```python
from build123d import *

# Parameters (mm, degrees)
SKETCH1_R           = 0.9
BOSS_EXTRUDE1_DEPTH = 5
SKETCH2_R           = 2.5
BOSS_EXTRUDE2_DEPTH = 1
DOME1_FACE_RADIUS   = 2.5
DOME1_HEIGHT        = 0.5
SKETCH3_W           = 1.125
SKETCH3_H           = 0.75
SKETCH3_W_2         = 0.75
SKETCH3_H_2         = 1.125
CUT_EXTRUDE1_DEPTH  = 0.75


with BuildPart() as part:
    # Sketch1 → Boss-Extrude1 (new body)
    with BuildSketch(Plane(origin=(0, 0, 0), x_dir=(1, 0, 0), z_dir=(0, 1, 0))):
        Circle(SKETCH1_R)
    extrude(amount=BOSS_EXTRUDE1_DEPTH)

    # Sketch2 → Boss-Extrude2 (add)
    with BuildSketch(Plane(origin=(0, 5, 0), x_dir=(1, 0, 0), z_dir=(0, 1, 0))):
        Circle(SKETCH2_R)
    extrude(amount=BOSS_EXTRUDE2_DEPTH)

    # Dome1: a dome of height H over a round flat face of radius A is a cap of a sphere of radius (A * A + H * H) / (2 * H)
    dome1_r = (DOME1_FACE_RADIUS * DOME1_FACE_RADIUS + DOME1_HEIGHT * DOME1_HEIGHT) / (2 * DOME1_HEIGHT)
    dome1_base = Plane((0, 6, 0), z_dir=(0, 1, 0))
    with Locations(dome1_base.offset(DOME1_HEIGHT - dome1_r)):
        dome1_ball = Sphere(dome1_r, mode=Mode.PRIVATE)
    add(split(dome1_ball, bisect_by=dome1_base, keep=Keep.TOP, mode=Mode.PRIVATE))

    # Sketch3 → Cut-Extrude1 (cut)
    with BuildSketch(Plane(origin=(0, 6.5, 0), x_dir=(1, 0, 0), z_dir=(0, 1, 0))):
        with Locations((-0.9375, 0)):
            Rectangle(SKETCH3_W, SKETCH3_H)
        Rectangle(SKETCH3_W_2, SKETCH3_H)
        with Locations((0, 0.9375)):
            Rectangle(SKETCH3_W_2, SKETCH3_H_2)
        with Locations((0.9375, 0)):
            Rectangle(SKETCH3_W, SKETCH3_H)
        with Locations((0, -0.9375)):
            Rectangle(SKETCH3_W_2, SKETCH3_H_2)
    extrude(amount=-CUT_EXTRUDE1_DEPTH, mode=Mode.SUBTRACT)


solid = part.part
```
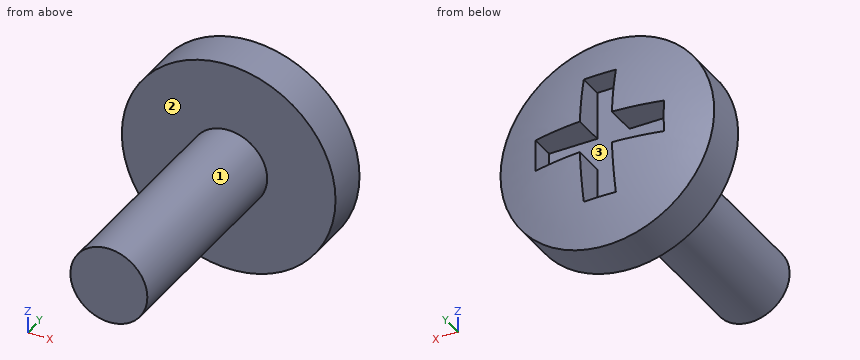
Geometry: final body of the model. Coordinates: model frame, mm. Face numbers are marked on the shaded views. Give positions to 0.01 mm unless a question says otherwise; leave off trailing zeros. Loops run counter-clockwise (first coordinate to the right, second up) from the corner with the lowest first, then second, coordinate; pieces in that order, holes last. Notation, with made-up numbers: (-28, -15.5) - (9, -15.5) arc R14 ccw to (9, -11.5) - close; hole circle Ø11 at (57, 39.25). An arc over 180 degrees is marked (long way). Answer as CSV lines item,"result". Start each with the question number.
(1) Pin query (flat end, axial travel): P1, Ø1, axis at x = -1.5, z = 0.5, coming from the -Y side; P2, Ø1, axis at x = 1, y = 2.5, coming from the +Z side; P3, Ø2, axis at x = -1, y = 3, coming from the -Z side. Return the tip coordinate at first contact, or that it passes through.
(2) Section query A-A (x = 0). Output: boundary loops of the cut face in (y, z).
(3) Mould query, pull axis X, two halves, no side actions, for the marked faces 1, 2 and 3. Classes: +X half, -X half, draft (parallel to the pull), parting line (faces both ways), or undercut.
(4) Section query B-B (z = 0). Output: boundary loops of the cut face in (x, y), and give its area (3 significant figures).
(5) Section query C-C (y = 3.5). Output: boundary loops of the cut face in (x, z), and give its area (3 significant figures).
(6) Ray query, line 1 along Y through (x, z) = (-0.2, -1.2); line 2 along Y through (x, z) = (-0.2, -0.55); line 3 along X through (y, z) = (1.25, -0.05). Return the intervals inside material, ascending. Write a range as [from, to].
Worked answers:
1,P1,"stops at y = 5"
1,P2,"stops at z = 0.75"
1,P3,"stops at z = -0.9"
2,outline,"(0, -0.9) - (5, -0.9) - (5, -2.5) - (6, -2.5) arc R6.5 ccw to (6.32, -1.5) - (5.75, -1.5) - (5.75, 1.5) - (6.32, 1.5) arc R6.5 ccw to (6, 2.5) - (5, 2.5) - (5, 0.9) - (0, 0.9) - close"
3,face 1,"parting line"
3,face 2,"draft"
3,face 3,"undercut"
4,outline,"(-2.5, 5) - (-0.9, 5) - (-0.9, 0) - (0.9, 0) - (0.9, 5) - (2.5, 5) - (2.5, 6) arc R6.5 ccw to (1.5, 6.32) - (1.5, 5.75) - (-1.5, 5.75) - (-1.5, 6.32) arc R6.5 ccw to (-2.5, 6) - close"
4,area,"13.6 mm^2"
5,outline,"circle Ø1.8 at (0, 0)"
5,area,"2.54 mm^2"
6,line 1,"y = [5, 5.75]"
6,line 2,"y = [0, 5.75]"
6,line 3,"x = [-0.9, 0.9]"
